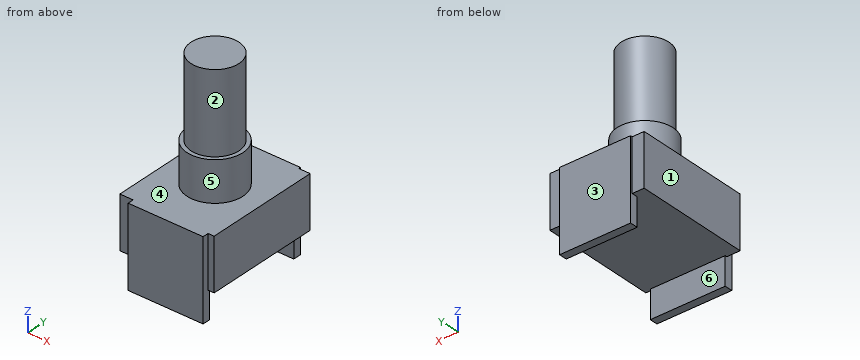
from build123d import *

# Parameters (mm, degrees)
SKETCH012_W   = 11.8
SKETCH012_H   = 14.5
PAD009_DEPTH  = 6.5
SKETCH013_R   = 3.5
PAD010_DEPTH  = 5
SKETCH014_R   = 3
PAD011_DEPTH  = 15
SKETCH015_W   = 8.880223
SKETCH015_H   = 1
SKETCH015_W_2 = 9.377943
PAD012_DEPTH  = 10


with BuildPart() as part:
    # Sketch012 → Pad009 (new body)
    with BuildSketch(Plane.XY):
        Rectangle(SKETCH012_W, SKETCH012_H)
    extrude(amount=-PAD009_DEPTH)

    # Sketch013 → Pad010 (join)
    with BuildSketch(Plane.XY):
        Circle(SKETCH013_R)
    extrude(amount=PAD010_DEPTH)

    # Sketch014 → Pad011 (join)
    with BuildSketch(Plane.XY):
        Circle(SKETCH014_R)
    extrude(amount=PAD011_DEPTH)

    # Sketch015 → Pad012 (join)
    with BuildSketch(Plane.XY):
        with Locations((0.034908, 7)):
            Rectangle(SKETCH015_W, SKETCH015_H)
        with Locations((0.447315, -7.5)):
            Rectangle(SKETCH015_W_2, SKETCH015_H)
    extrude(amount=-PAD012_DEPTH)


solid = part.part
Can you work these out from the model? Positions are in its coordinate system, mm. Face numbers are marked on the shaded views. A direction names the side the tool comes from. Give positions to 0.01 mm unless a question says otherwise; leave off trailing zeros. Loops run counter-clockwise (first coordinate to the right, second up) from the corner with the lowest first, then second, coordinate; pieces in that order, holes last. Notation, with made-up numbers: M 73,-7.5 L 131,-7.5 A10 cw 131,2.5 Z; hole C -18.75,7.5 d9. An arc over 180 degrees is marked long. One line per item, written item: value.
1) Imagine slicing it at A-A on x = 0. Write out the boundary of the cut face in (y, z).
Geometry check:
outline: M -8,-10 L -7,-10 L -7,-6.5 L 6.5,-6.5 L 6.5,-10 L 7.5,-10 L 7.5,0 L 3.5,0 L 3.5,5 L 3,5 L 3,15 L -3,15 L -3,5 L -3.5,5 L -3.5,0 L -8,0 Z
2) On a 3-axis mill with a long thin cutter (end or side, diameter ignored), from which of +Z, -Z, +X, -X, +Y, -Y can I reach the whole of each face in a straight line? I mean the marked faces 1 and 2. Say none if no direction works.
Geometry check:
face 1: +Z, -Z, -X, +Y, -Y
face 2: +Z
3) I'm going to push flat-ended pins straight in: pin 1 (0.5 mm diameter, centred on y = 7, z = -7, fed in from -X); pin 2 (0.7 mm diameter, centred on x = 5, z = -2.5, fed in from +Y); pin 3 (0.8 mm diameter, centred on y = 7, z = -7, fed in from +X) (3 decimals). Where does each tip first touch, or does it pass through?
Geometry check:
pin 1: stops at x = -4.41
pin 2: stops at y = 7.25
pin 3: stops at x = 4.475
4) Please list where these lines run through material, in increasing order: line 1 (Y direction, x = -2.25, z = -8.5); line 2 (Z direction, x = -5.5, y = 4.5); line 3 (Z direction, x = -3, y = 0.5).
Geometry check:
line 1: y = -8 to -7, 6.5 to 7.5
line 2: z = -6.5 to 0
line 3: z = -6.5 to 5
5) Imagine slicing it at B-B on y = 0. Write out the boundary of the cut face in (x, z).
Geometry check:
outline: M -5.9,-6.5 L 5.9,-6.5 L 5.9,0 L 3.5,0 L 3.5,5 L 3,5 L 3,15 L -3,15 L -3,5 L -3.5,5 L -3.5,0 L -5.9,0 Z
6) Imagine slicing it at C-C on z = 5.75. Write out the boundary of the cut face in (x, y).
Geometry check:
outline: C 0,0 d6
7) Imagine slicing it at D-D on x = 1.5. Write out the boundary of the cut face in (y, z).
Geometry check:
outline: M -8,-10 L -7,-10 L -7,-6.5 L 6.5,-6.5 L 6.5,-10 L 7.5,-10 L 7.5,0 L 3.16,0 L 3.16,5 L 2.6,5 L 2.6,15 L -2.6,15 L -2.6,5 L -3.16,5 L -3.16,0 L -8,0 Z
8) Thinking about a two-plate mould opening in Y: for the marked faces 3, 4, 5 and 6, which applies, +Y half, -Y half, draft (parallel to the pull), parting line (faces both ways), or undercut?
Geometry check:
face 3: +Y half
face 4: draft
face 5: parting line
face 6: undercut
